Job drawing, mm, ordinate dimensions from the low corner. One solid piece. Coordinates: 2 decimals unless noted, no trailing zeros. Order: outer loops, then holes, each group sorted by start corner. A loop starts at its lowest first (then second) coordinate and runs counter-clockwise, first axis right, second up. Notation, with made-up numbers: (49, 48) -> (80, 48) arc R29 cw to (80, 87) -> close; hole circle Ø8 at (78.25, -27.75). An arc over 180 degrees is marked (long way). Use CSV: the item, a comma, the result in double quotes. Start each with the question number.
(1) Pull direction Z, two halves, no side cores. Call the marked faces 1, 2 and 3: pulls with the +Z half, pulls with the -Z half, needs draft (parallel to the pull), parting line crosses it, or undercut.
(2) Cut at C-C on x = 8.35. Write the cut outline in (y, z).
(3) Cut at D-D on y = 2.5. Write the cut outline in (x, z).
(4) Cut at B-B on z = 12.85. Write the cut outline in (x, y).
(5) Pin check, flat tips, straight feed: pin 1 Ø1 at (y, z) = (1, 14) entering from -X; pin 2 Ø1 at (x, y) = (18.5, 1.5) entering from -Z; pin 3 Ø3 at (x, y) = (16, 1) entering from -Z. Stop position of each tip, or through.
(6) Cut at A-A on x = 12.85. Write the cut outline in (y, z).
(7) Probe L1, parallel to Z at x = 17.25, y = 1.65 (1 decimal); L2, parallel to X at y = 0.5, z = 5.75; L3, parallel to Z at x = 16.5, y = 2.2. List the from-to ranges inside material, lowest first.
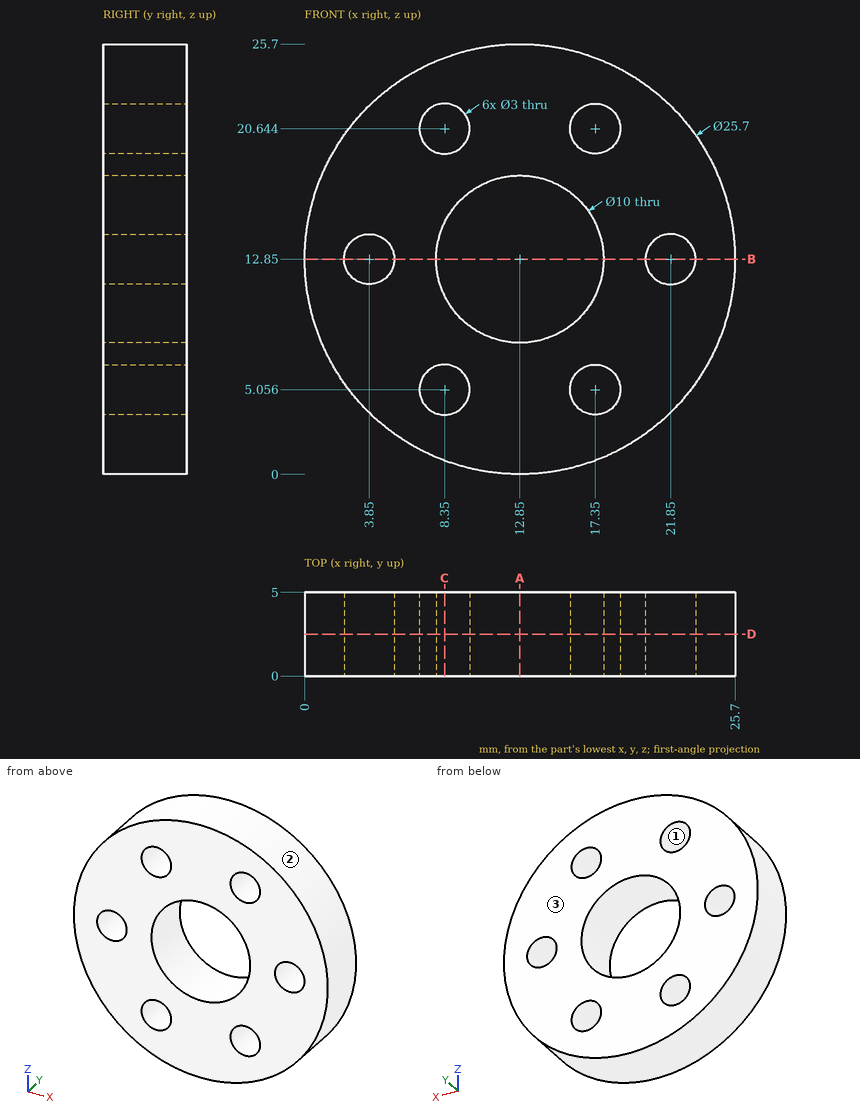
Outcome:
1,face 1,"undercut"
1,face 2,"parting line crosses it"
1,face 3,"needs draft"
2,outline,"(0, 0.81) -> (5, 0.81) -> (5, 3.56) -> (0, 3.56) -> close; (0, 6.56) -> (5, 6.56) -> (5, 10.67) -> (0, 10.67) -> close; (0, 15.03) -> (5, 15.03) -> (5, 19.14) -> (0, 19.14) -> close; (0, 22.14) -> (5, 22.14) -> (5, 24.89) -> (0, 24.89) -> close"
3,outline,"circle Ø25.7 at (12.85, 12.85); hole circle Ø3 at (3.85, 12.85); hole circle Ø3 at (8.35, 5.06); hole circle Ø3 at (8.35, 20.64); hole circle Ø10 at (12.85, 12.85); hole circle Ø3 at (17.35, 5.06); hole circle Ø3 at (17.35, 20.64); hole circle Ø3 at (21.85, 12.85)"
4,outline,"(0, 0) -> (2.35, 0) -> (2.35, 5) -> (0, 5) -> close; (5.35, 0) -> (7.85, 0) -> (7.85, 5) -> (5.35, 5) -> close; (17.85, 0) -> (20.35, 0) -> (20.35, 5) -> (17.85, 5) -> close; (23.35, 0) -> (25.7, 0) -> (25.7, 5) -> (23.35, 5) -> close"
5,pin 1,"x = 0.02"
5,pin 2,"z = 1.08"
5,pin 3,"z = 0.11"
6,outline,"(0, 0) -> (5, 0) -> (5, 7.85) -> (0, 7.85) -> close; (0, 17.85) -> (5, 17.85) -> (5, 25.7) -> (0, 25.7) -> close"
7,L1,"0.8 to 3.6, 6.6 to 10.5, 15.2 to 19.1, 22.1 to 24.9"
7,L2,"2.14 to 7.02, 9.68 to 16.02, 18.68 to 23.56"
7,L3,"0.53 to 3.82, 6.29 to 9.43, 16.27 to 19.41, 21.88 to 25.17"
